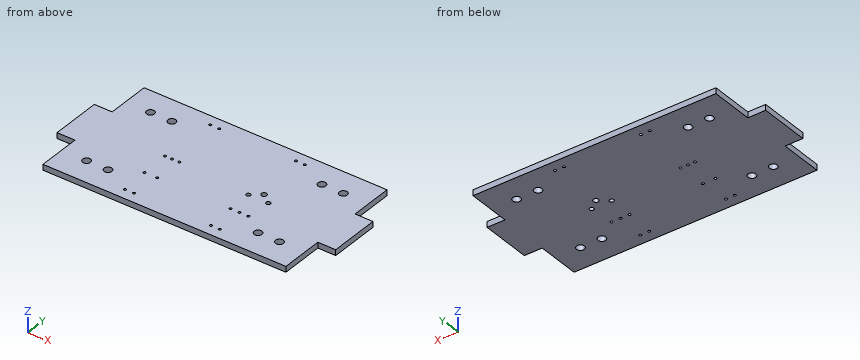
```python
from build123d import *

# Parameters (mm, degrees)
F0_W     = 68
F0_H     = 12
F0_W_2   = 5
F0_H_2   = 14
F1_DEPTH = 1.6
F4_R     = 0.35
F5_R     = 0.35
F6_R     = 0.35
F2_R     = 0.35
F7_DEPTH = 4
F8_R     = 1.1
F9_DEPTH = 25


with BuildPart() as f1:
    # F0 (on Top) → F1 (new body)
    with BuildSketch(Plane.XY):
        with Locations((41.3172904253, 1.6970097786)):
            Rectangle(F0_W, F0_H)
        with Locations((4.8172904253, 14.6970097786)):
            Rectangle(F0_W_2, F0_H_2)
        with Locations((41.3172904253, 14.6970097786)):
            Rectangle(F0_W, F0_H_2)
        with Locations((77.8172904253, 14.6970097786)):
            Rectangle(F0_W_2, F0_H_2)
        with Locations((41.3172904253, 27.6970097786)):
            Rectangle(F0_W, F0_H)
    extrude(amount=F1_DEPTH)

    # F4 (on face) + F5 (on face) + F6 (on face) + F3 (on face) + F2 (on face) → F7 (cut)
    with BuildSketch(Plane.XY.offset(1.6)):
        with Locations((51.6172904253, 6.6970097786)):
            Circle(F4_R)
        with Locations((56.6172904253, 6.6970097786)):
            Circle(F4_R)
        with Locations((54.1172904253, 6.6970097786)):
            Circle(F4_R)
    with BuildSketch(Plane.XY.offset(1.6)):
        with Locations((28.0672904253, -1.3029902214)):
            Circle(F5_R)
        with Locations((30.5672904253, -1.3029902214)):
            Circle(F5_R)
        with Locations((52.0672904253, -1.3029902214)):
            Circle(F5_R)
        with Locations((54.5672904253, -1.3029902214)):
            Circle(F5_R)
        with Locations((54.5672904253, 30.6970097786)):
            Circle(F5_R)
        with Locations((52.0672904253, 30.6970097786)):
            Circle(F5_R)
        with Locations((30.5672904253, 30.6970097786)):
            Circle(F5_R)
        with Locations((28.0672904253, 30.6970097786)):
            Circle(F5_R)
    with BuildSketch(Plane.XY.offset(1.6)):
        with Locations((27.5672904253, 6.6970097786)):
            Circle(F6_R)
        with Locations((31.0672904253, 6.6970097786)):
            Circle(F6_R)
    with BuildSketch(Plane.XY.offset(1.6)):
        with BuildLine():
            Line((54.8172904253, 15.4470097786), (53.8172904253, 15.4470097786))
            ThreePointArc((53.8172904253, 15.4470097786), (53.640513733, 15.5202330803), (53.5672904253, 15.6970097701))
            ThreePointArc((53.5672904253, 15.6970097701), (54.3172904296, 14.9470097786), (55.0672904253, 15.6970097786))
            ThreePointArc((55.0672904253, 15.6970097786), (54.9940671206, 15.5202330833), (54.8172904253, 15.4470097786))
        make_face()
        with BuildLine():
            ThreePointArc((53.5672904253, 15.6970097701), (53.640513733, 15.5202330803), (53.8172904253, 15.4470097786))
            Line((53.8172904253, 15.4470097786), (54.8172904253, 15.4470097786))
            ThreePointArc((54.8172904253, 15.4470097786), (54.9940671206, 15.5202330833), (55.0672904253, 15.6970097786))
            ThreePointArc((55.0672904253, 15.6970097786), (54.9940671206, 15.8737864739), (54.8172904253, 15.9470097786))
            Line((54.8172904253, 15.9470097786), (53.8172904253, 15.9470097786))
            ThreePointArc((53.8172904253, 15.9470097786), (53.640513727, 15.8737864709), (53.5672904253, 15.6970097701))
        make_face()
        with BuildLine():
            ThreePointArc((55.0672904253, 15.6970097786), (54.317290421, 16.4470097786), (53.5672904253, 15.6970097701))
            ThreePointArc((53.5672904253, 15.6970097701), (53.640513727, 15.8737864709), (53.8172904253, 15.9470097786))
            Line((53.8172904253, 15.9470097786), (54.8172904253, 15.9470097786))
            ThreePointArc((54.8172904253, 15.9470097786), (54.9940671206, 15.8737864739), (55.0672904253, 15.6970097786))
        make_face()
        with BuildLine():
            Line((51.1672904253, 13.7970097786), (51.8672904253, 13.7970097786))
            ThreePointArc((51.8672904253, 13.7970097786), (52.0440671206, 13.7237864739), (52.1172904253, 13.5470097786))
            ThreePointArc((52.1172904253, 13.5470097786), (51.5172904253, 14.1470097786), (50.9172904253, 13.5470097786))
            ThreePointArc((50.9172904253, 13.5470097786), (50.99051373, 13.7237864739), (51.1672904253, 13.7970097786))
        make_face()
        with BuildLine():
            ThreePointArc((52.1172904253, 13.5470097786), (52.0440671206, 13.7237864739), (51.8672904253, 13.7970097786))
            Line((51.8672904253, 13.7970097786), (51.1672904253, 13.7970097786))
            ThreePointArc((51.1672904253, 13.7970097786), (50.99051373, 13.7237864739), (50.9172904253, 13.5470097786))
            ThreePointArc((50.9172904253, 13.5470097786), (50.99051373, 13.3702330833), (51.1672904253, 13.2970097786))
            Line((51.1672904253, 13.2970097786), (51.8672904253, 13.2970097786))
            ThreePointArc((51.8672904253, 13.2970097786), (52.0440671206, 13.3702330833), (52.1172904253, 13.5470097786))
        make_face()
        with BuildLine():
            ThreePointArc((50.9172904253, 13.5470097786), (51.5172904253, 12.9470097786), (52.1172904253, 13.5470097786))
            ThreePointArc((52.1172904253, 13.5470097786), (52.0440671206, 13.3702330833), (51.8672904253, 13.2970097786))
            Line((51.8672904253, 13.2970097786), (51.1672904253, 13.2970097786))
            ThreePointArc((51.1672904253, 13.2970097786), (50.99051373, 13.3702330833), (50.9172904253, 13.5470097786))
        make_face()
        with BuildLine():
            Line((56.7672904253, 13.2970097786), (57.4672904253, 13.2970097786))
            ThreePointArc((57.4672904253, 13.2970097786), (57.6440671206, 13.3702330833), (57.7172904253, 13.5470097786))
            ThreePointArc((57.7172904253, 13.5470097786), (57.6440671206, 13.7237864739), (57.4672904253, 13.7970097786))
            Line((57.4672904253, 13.7970097786), (56.7672904253, 13.7970097786))
            ThreePointArc((56.7672904253, 13.7970097786), (56.59051373, 13.7237864739), (56.5172904253, 13.5470097786))
            ThreePointArc((56.5172904253, 13.5470097786), (56.59051373, 13.3702330833), (56.7672904253, 13.2970097786))
        make_face()
        with BuildLine():
            ThreePointArc((57.7172904253, 13.5470097786), (57.6440671206, 13.3702330833), (57.4672904253, 13.2970097786))
            Line((57.4672904253, 13.2970097786), (56.7672904253, 13.2970097786))
            ThreePointArc((56.7672904253, 13.2970097786), (56.59051373, 13.3702330833), (56.5172904253, 13.5470097786))
            ThreePointArc((56.5172904253, 13.5470097786), (57.1172904253, 12.9470097786), (57.7172904253, 13.5470097786))
        make_face()
        with BuildLine():
            ThreePointArc((57.4672904253, 13.7970097786), (57.6440671206, 13.7237864739), (57.7172904253, 13.5470097786))
            ThreePointArc((57.7172904253, 13.5470097786), (57.1172904253, 14.1470097786), (56.5172904253, 13.5470097786))
            ThreePointArc((56.5172904253, 13.5470097786), (56.59051373, 13.7237864739), (56.7672904253, 13.7970097786))
            Line((56.7672904253, 13.7970097786), (57.4672904253, 13.7970097786))
        make_face()
    with BuildSketch(Plane.XY.offset(1.6)):
        with Locations((27.3172904253, 14.6970097786)):
            Circle(F2_R)
        with Locations((29.3172904253, 14.6970097786)):
            Circle(F2_R)
        with Locations((31.3172904253, 14.6970097786)):
            Circle(F2_R)
    extrude(amount=-F7_DEPTH, mode=Mode.SUBTRACT)

    # F8 (on face) → F9 (cut)
    with BuildSketch(Plane.XY.offset(1.6)):
        with Locations((62.3172904253, 26.6970097786)):
            Circle(F8_R)
        with Locations((20.3172904253, 26.6970097786)):
            Circle(F8_R)
        with Locations((68.3172904253, 2.6970097786)):
            Circle(F8_R)
        with Locations((14.3172904253, 2.6970097786)):
            Circle(F8_R)
        with Locations((62.3172904253, 2.6970097786)):
            Circle(F8_R)
        with Locations((20.3172904253, 2.6970097786)):
            Circle(F8_R)
        with Locations((68.3172904253, 26.6970097786)):
            Circle(F8_R)
        with Locations((14.3172904253, 26.6970097786)):
            Circle(F8_R)
    extrude(amount=-F9_DEPTH, mode=Mode.SUBTRACT)


solid = f1.part
```
Geometry: final body of the model. Coordinates: model frame, mm. Coordinates: 2 decimals unless noted, no trailing zeros. Loops run counter-clockwise (first coordinate to the right, second up) from the corner with the lowest first, then second, coordinate; pieces in that order, holes last. Notation, with made-up numbers: (85, 14) -> (111, 14) arc R12 cw to (111, 33) -> close; hole circle Ø6 at (-14, 35). An arc over 180 degrees is marked (long way). Use a Markdown table: item, result. Add a question column.
(1) Pin query (flat end, axial travel): pin 1 Ø0.8 at (y, z) = (4, 0.5) entering from -X; pin 2 Ø1.4 at (x, y) = (51.52, 13.55) entering from +Z; pin 3 Ø0.8 at (y, z) = (1, 0.5) entering from +X. Return the tip coordinate at first contact, or that it passes through.
(2) Section query B-B, the plane z = 1.15. State how many separate pieces and enclosed holes the cut face has, plus the area to 3 significant figures.
(3) Line query: line 1 along X through (y, z) = (3.5, 0.65); line 2 along X through (y, z) = (2, 0.3); line 3 along X through (y, z) = (4, 0.35). Output: solid intervals per line, ascending.
(4) Section query A-A, the plane y = 22.5. Return loops of the section in (x, z), plus the area to 3 significant figures.
Answer:
| question | item | result |
|---|---|---|
| 1 | pin 1 | stops at x = 7.32 |
| 1 | pin 2 | stops at z = 1.6 |
| 1 | pin 3 | stops at x = 75.32 |
| 2 | separate pieces | 1 |
| 2 | enclosed holes | 27 |
| 2 | area | 2,680 mm^2 |
| 3 | line 1 | x = 7.32 to 13.57, 15.07 to 19.57, 21.07 to 61.57, 63.07 to 67.57, 69.07 to 75.32 |
| 3 | line 2 | x = 7.32 to 13.47, 15.17 to 19.47, 21.17 to 61.47, 63.17 to 67.47, 69.17 to 75.32 |
| 3 | line 3 | x = 7.32 to 75.32 |
| 4 | outline | (7.32, 0) -> (75.32, 0) -> (75.32, 1.6) -> (7.32, 1.6) -> close |
| 4 | area | 109 mm^2 |
